from build123d import *

# Parameters (mm, degrees)
BOSS_EXTRUDE1_DEPTH            = 1.5
M5_CLEARANCE_HOLE1_D           = 5.5
M5_CLEARANCE_HOLE1_CSINK_D     = 5.55
M5_CLEARANCE_HOLE1_CSINK_ANGLE = 90


with BuildPart() as part:
    # Sketch1 → Boss-Extrude1 (new, symmetric)
    with BuildSketch(Plane(origin=(0, 0, 0), x_dir=(1, 0, 0), z_dir=(0, 1, 0))):
        Polygon((100, 15), (97, 15), (85.5, 15), (85.5, 12), (76.5, 12), (76.5, 15), (67.5, 15), (67.5, 12), (58.5, 12), (58.5, 15), (49.5, 15), (49.5, 12), (40.5, 12), (40.5, 15), (31.5, 15), (31.5, 12), (22.5, 12), (22.5, 15), (13.5, 15), (13.5, 12), (4.5, 12), (4.5, 15), (-4.5, 15), (-4.5, 12), (-13.5, 12), (-13.5, 15), (-22.5, 15), (-22.5, 12), (-31.5, 12), (-31.5, 15), (-40.5, 15), (-40.5, 12), (-49.5, 12), (-49.5, 15), (-58.5, 15), (-58.5, 12), (-67.5, 12), (-67.5, 15), (-76.5, 15), (-76.5, 12), (-85.5, 12), (-85.5, 15), (-97, 15), (-100, 15), (-100, 12), (-100, 4.5), (-97, 4.5), (-97, -4.5), (-100, -4.5), (-100, -12), (-100, -15), (-97, -15), (-85.5, -15), (-85.5, -12), (-76.5, -12), (-76.5, -15), (-67.5, -15), (-67.5, -12), (-58.5, -12), (-58.5, -15), (-49.5, -15), (-49.5, -12), (-40.5, -12), (-40.5, -15), (-31.5, -15), (-31.5, -12), (-22.5, -12), (-22.5, -15), (-13.5, -15), (-13.5, -12), (-4.5, -12), (-4.5, -15), (4.5, -15), (4.5, -12), (13.5, -12), (13.5, -15), (22.5, -15), (22.5, -12), (31.5, -12), (31.5, -15), (40.5, -15), (40.5, -12), (49.5, -12), (49.5, -15), (58.5, -15), (58.5, -12), (67.5, -12), (67.5, -15), (76.5, -15), (76.5, -12), (85.5, -12), (85.5, -15), (97, -15), (100, -15), (100, -12), (100, -4.5), (97, -4.5), (97, 4.5), (100, 4.5), (100, 12), align=None)
    extrude(amount=BOSS_EXTRUDE1_DEPTH, both=True)

    # M5 Clearance Hole1 (through all)
    with Locations(Plane(origin=(0, 1.5, 0), x_dir=(1, 0, 0), z_dir=(0, 1, 0))):
        with Locations((54, 4.5), (-79, 4.5), (-54, 4.5), (79, 4.5)):
            CounterSinkHole(M5_CLEARANCE_HOLE1_D / 2, M5_CLEARANCE_HOLE1_CSINK_D / 2, counter_sink_angle=M5_CLEARANCE_HOLE1_CSINK_ANGLE)


solid = part.part
Can you work these out from the model? Positions are in its coordinate system, mm. Give positions to 0.01 mm unless a question says otherwise; leave off trailing zeros. Loops run counter-clockwise (first coordinate to the right, second up) from the corner with the lowest first, then second, coordinate; pieces in that order, holes last. Notation, with made-up numbers: (26, 83) -> (34, 83) arc R15 ccw to (34, 100) -> close; hole circle Ø1 at (-20.75, -13.5). An arc over 180 degrees is marked (long way). Write item = value, one per line.
1) Will this pin go through, and if not, where does the flat tip stop? pin 1 (0.9 mm diameter, centred on x = -27, y = -0.5, fed in from -Z).
Check result:
pin_1 = -12
2) I need wall thicknesses on L1, parallel to Z at x = -54, y = 0.3; L2, parallel to Z at x = -79, y = 0.1; L3, parallel to X at y = 1.25, z = -5. Which ranges of each line are inside material? Lowest first, please. Write a range as from..to.
Check result:
L1 = -15..-7.25, -1.75..15
L2 = -12..-7.25, -1.75..12
L3 = -100..-81.7, -76.3..-56.7, -51.3..51.3, 56.7..76.3, 81.7..100
3) Suppose I cut it at B-B on y = -0.4. Give the number of separate pieces and of enclosed holes in the cut face, then the cut area to 3 significant figures.
Check result:
separate_pieces = 1
enclosed_holes = 4
area = 5,310 mm2
4) Suppose I cut it at C-C on x = -54. Write out the boundary of the cut face in (y, z) (3 decimals).
Check result:
outline = (-1.5, -15) -> (1.5, -15) -> (1.5, -7.275) -> (1.475, -7.25) -> (-1.5, -7.25) -> close; (-1.5, -1.75) -> (1.475, -1.75) -> (1.5, -1.725) -> (1.5, 15) -> (-1.5, 15) -> close
5) Suppose I cut it at A-A on x = 79. Write out the boundary of the cut face in (y, z) (3 decimals).
Check result:
outline = (-1.5, -12) -> (1.5, -12) -> (1.5, -7.275) -> (1.475, -7.25) -> (-1.5, -7.25) -> close; (-1.5, -1.75) -> (1.475, -1.75) -> (1.5, -1.725) -> (1.5, 12) -> (-1.5, 12) -> close
6) Thinking about a two-plate mould opening in Z: for faces 1 (the flat face through (-1, 1.5, 0)), 2 (the cylindrical face through (81.747, -0.033, -4.621)), 3 (the cylindrical face through (-51.253, -0.033, -4.621)), which applies, released by +Z, released by -Z, zero draft, split by the parting line, or undercut?
Check result:
face_1 = zero draft
face_2 = undercut
face_3 = undercut
7) Suppose I cut it at D-D on z = 1.25. Write out the boundary of the cut face in (x, y).
Check result:
outline = (-97, -1.5) -> (97, -1.5) -> (97, 1.5) -> (-97, 1.5) -> close
